Could you check a few things on this model? Use its own coordinates, in mm. Give positions to 0.01 mm unless a question says otherwise; leave off trailing zeros. Loops run counter-clockwise (first coordinate to the right, second up) from the corner with the lowest first, then second, coordinate; pieces in that order, holes last. Notation, with made-up numbers: (55.5, -27.75) - (65.5, -27.75) arc R11 ccw to (65.5, -22.75) - close; hole circle Ø8 at (56, -15.75). An arc over 180 degrees is marked (long way). One line per item, written item: value. Start each with the question number.
Q1. I'm going to push flat-ended pins straight in: P1, Ø1.5, axis at y = -3, z = -30, coming from the +X side; P2, Ø1.5, axis at y = -3.5, z = -52, coming from the +X side; P3, Ø2.5, axis at y = -1.5, z = -53.5, coming from the -X side. Where does each tip first touch, or does it pass through?
Q2. I want a section at A-A (x = 125). Please give me the cut outline in (y, z).
Q3. If I drill on line 1 (X direction, y = -4.45, z = 40.5); line 2 (Z direction, x = 125, y = -3.25); line 3 (X direction, y = -2.05, z = -10.5), over which ranges is the centre line in solid material (lowest first)? Write a range as from..to.
Q4. I want a section at C-C (x = -158). Please give me the cut outline in (y, z).
Q5. I want a section at B-B (y = -1.65). Please give me the cut outline in (x, z), then the cut area to 3 significant figures.
```python
from build123d import *

# Parameters (mm, degrees)
F0_R     = 12.5
F0_W     = 98
F0_H     = 5
F0_W_2   = 5
F0_H_2   = 50
F0_H_3   = 100
F1_DEPTH = 5


with BuildPart() as f1:
    # F0 (on Front) → F1 (new body)
    with BuildSketch(Plane.XZ):
        Polygon((147, -50), (245, -50), (245, 0), (245, 50), (130, 50), (130, 40), (125, 40), (120, 40), (120, 50), (5, 50), (5, -50), (49, -50), align=None)
        with Locations((125, 0)):
            Circle(F0_R, mode=Mode.SUBTRACT)
        with Locations((98, -52.5)):
            Rectangle(F0_W, F0_H)
        with Locations((247.5, 25)):
            Rectangle(F0_W_2, F0_H_2)
        with Locations((2.5, 0)):
            Rectangle(F0_W_2, F0_H_3)
        with Locations((-2.5, 0)):
            Rectangle(F0_W_2, F0_H_3)
        with BuildLine():
            Line((-113.4615384615, -4.8076923077), (-5, -50))
            Line((-5, -50), (-5, 50))
            Line((-5, 50), (-113.4615384615, 4.8076923077))
            ThreePointArc((-113.4615384615, 4.8076923077), (-112.7427415539, 2.4514516892), (-112.5, 0))
            ThreePointArc((-112.5, 0), (-112.7427415539, -2.4514516892), (-113.4615384615, -4.8076923077))
        make_face()
        with BuildLine():
            Line((-49, -50), (-5, -50))
            Line((-5, -50), (-113.4615384615, -4.8076923077))
            ThreePointArc((-113.4615384615, -4.8076923077), (-125, -12.5), (-136.5384615385, -4.8076923077))
            Line((-136.5384615385, -4.8076923077), (-245, -50))
            Line((-245, -50), (-147, -50))
            Line((-147, -50), (-49, -50))
        make_face()
        with Locations((-98, -52.5)):
            Rectangle(F0_W, F0_H)
        with BuildLine():
            Line((-113.4615384615, 4.8076923077), (-5, 50))
            Line((-5, 50), (-120, 50))
            Line((-120, 50), (-120, 40))
            Line((-120, 40), (-125, 40))
            Line((-125, 40), (-125, 12.5))
            ThreePointArc((-125, 12.5), (-118.0662475472, 10.4006286792), (-113.4615384615, 4.8076923077))
        make_face()
        with BuildLine():
            Line((-245, -50), (-136.5384615385, -4.8076923077))
            ThreePointArc((-136.5384615385, -4.8076923077), (-137.5, 0), (-136.5384615385, 4.8076923077))
            Line((-136.5384615385, 4.8076923077), (-245, 50))
            Line((-245, 50), (-245, 0))
            Line((-245, 0), (-245, -50))
        make_face()
        with BuildLine():
            ThreePointArc((-136.5384615385, 4.8076923077), (-131.9337524528, 10.4006286792), (-125, 12.5))
            Line((-125, 12.5), (-125, 40))
            Line((-125, 40), (-130, 40))
            Line((-130, 40), (-130, 50))
            Line((-130, 50), (-245, 50))
            Line((-245, 50), (-136.5384615385, 4.8076923077))
        make_face()
        with Locations((-247.5, 25)):
            Rectangle(F0_W_2, F0_H_2)
    extrude(amount=F1_DEPTH)


solid = f1.part
```
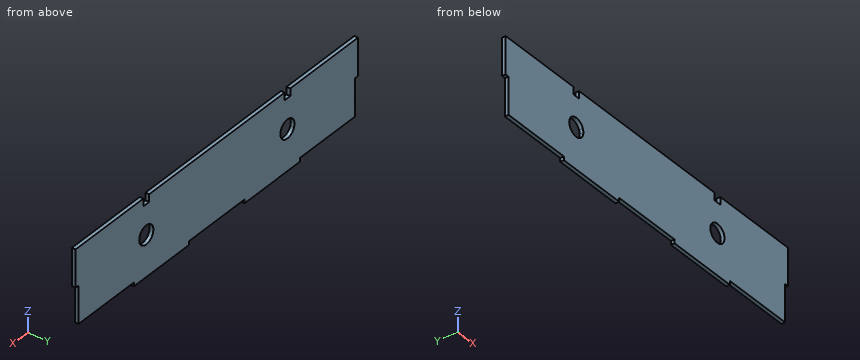
Worked answers:
1. P1: stops at x = 245
1. P2: stops at x = 147
1. P3: stops at x = -147
2. outline: (-5, -55) - (0, -55) - (0, -12.5) - (-5, -12.5) - close; (-5, 12.5) - (0, 12.5) - (0, 40) - (-5, 40) - close
3. line 1: x = -250..-130, -120..120, 130..250
3. line 2: z = -55..-12.5, 12.5..40
3. line 3: x = -245..-131.78, -118.22..118.22, 131.78..245
4. outline: (-5, -50) - (0, -50) - (0, 50) - (-5, 50) - close
5. outline: (-250, 0) - (-245, 0) - (-245, -50) - (-147, -50) - (-147, -55) - (-49, -55) - (-49, -50) - (49, -50) - (49, -55) - (147, -55) - (147, -50) - (245, -50) - (245, 0) - (250, 0) - (250, 50) - (130, 50) - (130, 40) - (120, 40) - (120, 50) - (-120, 50) - (-120, 40) - (-130, 40) - (-130, 50) - (-250, 50) - close; hole circle Ø25 at (-125, 0); hole circle Ø25 at (125, 0)
5. area: 49,300 mm²
